Input: part model. Units: mm. Frame: model coordinates. A direction names the side the tool comes from. Give positions to 0.01 mm unless a question says otherwise; leave off trailing zeros. Order: outer loops, then holes, each group sorted by start corner. A loop starts at its lowest first (then second) coordinate and runs counter-clockwise, first axis right, second up. Notation, with made-up numbers: (87.5, 67.5) -> (135.5, 67.5) arc R8 cw to (135.5, 80.5) -> close; hole circle Ø11 at (72, 13). An arc over 180 degrees is marked (long way). Use a Markdown table: item, result. Add a question column.
from build123d import *

# Parameters (mm, degrees)
SKIZZE1_R                                            = 52.5
AUFSATZ_LINEAR_AUSTRAGEN1_DEPTH                      = 10
SKIZZE2_R                                            = 40
AUFSATZ_LINEAR_AUSTRAGEN3_DEPTH                      = 5
SKIZZE5_OUTSIDE_W                                    = 136.85
SKIZZE5_OUTSIDE_H                                    = 136.85
SKIZZE5_OUTSIDE_R                                    = 35
SCHNITT_LINEAR_AUSTRAGEN1_DEPTH                      = 5
SKIZZE6_R                                            = 38
AUFSATZ_LINEAR_AUSTRAGEN4_DEPTH                      = 5
SCHNITT_LINEAR_START                                 = -5
SKIZZE7_R                                            = 34.75
SCHNITT_LINEAR_AUSTRAGEN2_DEPTH                      = 10
SKIZZE10_R                                           = 25
SCHNITT_LINEAR_AUSTRAGEN4_DEPTH                      = 10
STIRNSENKUNG_F_R_M5_ZYLINDERSCHRAUBE_MIT_D           = 5.5
STIRNSENKUNG_F_R_M5_ZYLINDERSCHRAUBE_MIT_CBORE_D     = 10
STIRNSENKUNG_F_R_M5_ZYLINDERSCHRAUBE_MIT_CBORE_DEPTH = 5.4
KREISMUSTER4_COUNT                                   = 6
SKIZZE16_R                                           = 39
SKIZZE16_R_2                                         = 38
O_RING_NUT_DEPTH                                     = 1
SKIZZE17_R                                           = 40.85
SKIZZE17_R_2                                         = 38
SCHNITT_LINEAR_AUSTRAGEN5_DEPTH                      = 1.45
VERRUNDUNG1_R                                        = 0.3


with BuildPart() as part:
    # Skizze1 → Aufsatz-Linear austragen1 (new body)
    with BuildSketch(Plane.XY):
        Circle(SKIZZE1_R)
    extrude(amount=AUFSATZ_LINEAR_AUSTRAGEN1_DEPTH)

    # Skizze2 → Aufsatz-Linear austragen3 (add)
    with BuildSketch(Plane.XY):
        Circle(SKIZZE2_R)
    extrude(amount=-AUFSATZ_LINEAR_AUSTRAGEN3_DEPTH)

    # Skizze5 outside → Schnitt-Linear austragen1 (cut)
    with BuildSketch(Plane.XY):
        Rectangle(SKIZZE5_OUTSIDE_W, SKIZZE5_OUTSIDE_H)
        Circle(SKIZZE5_OUTSIDE_R, mode=Mode.SUBTRACT)
    extrude(amount=-SCHNITT_LINEAR_AUSTRAGEN1_DEPTH, mode=Mode.SUBTRACT)

    # Skizze6 → Aufsatz-Linear austragen4 (add)
    with BuildSketch(Plane.XY):
        Circle(SKIZZE6_R)
    extrude(amount=-AUFSATZ_LINEAR_AUSTRAGEN4_DEPTH)

    # Skizze7 → Schnitt-Linear austragen2 (cut)
    with BuildSketch(Plane.XY.offset(SCHNITT_LINEAR_START)):
        Circle(SKIZZE7_R)
    extrude(amount=SCHNITT_LINEAR_AUSTRAGEN2_DEPTH, mode=Mode.SUBTRACT)

    # Skizze10 → Schnitt-Linear austragen4 (cut)
    with BuildSketch(Plane.XY):
        Circle(SKIZZE10_R)
    extrude(amount=SCHNITT_LINEAR_AUSTRAGEN4_DEPTH, mode=Mode.SUBTRACT)

    # Stirnsenkung f_r M5 Zylinderschraube mit (through all)
    with Locations(Plane.XY.offset(10)):
        with Locations((0, -44)):
            stirnsenkung_f_r_m5_zylinderschraube_mit = CounterBoreHole(STIRNSENKUNG_F_R_M5_ZYLINDERSCHRAUBE_MIT_D / 2, STIRNSENKUNG_F_R_M5_ZYLINDERSCHRAUBE_MIT_CBORE_D / 2, STIRNSENKUNG_F_R_M5_ZYLINDERSCHRAUBE_MIT_CBORE_DEPTH)

    # Kreismuster4: Stirnsenkung f_r M5 Zylinderschraube mit ×6 about axis
    kreismuster4_axis = Axis((0, 0, 0), (0, 0, 1))
    for i in range(1, KREISMUSTER4_COUNT):
        add(stirnsenkung_f_r_m5_zylinderschraube_mit.rotate(kreismuster4_axis, i * 360 / KREISMUSTER4_COUNT), mode=Mode.SUBTRACT)

    # Skizze16 → o ring nut (cut)
    with BuildSketch(Plane(origin=(0, 0, 0), x_dir=(-1, 0, 0), z_dir=(0, 0, -1))):
        Circle(SKIZZE16_R)
        with Locations(Location((0, 0, 0), (0, 0, 180))):  # turned: the seam where the file's is
            Circle(SKIZZE16_R_2, mode=Mode.SUBTRACT)
    extrude(amount=-O_RING_NUT_DEPTH, mode=Mode.SUBTRACT)

    # Skizze17 → Schnitt-Linear austragen5 (cut)
    with BuildSketch(Plane(origin=(0, 0, 0), x_dir=(-1, 0, 0), z_dir=(0, 0, -1))):
        Circle(SKIZZE17_R)
        with Locations(Location((0, 0, 0), (0, 0, 180))):  # turned: the seam where the file's is
            Circle(SKIZZE17_R_2, mode=Mode.SUBTRACT)
    extrude(amount=-SCHNITT_LINEAR_AUSTRAGEN5_DEPTH, mode=Mode.SUBTRACT)

    # Verrundung1
    verrundung1_edges = [part.edges().sort_by_distance(p)[0] for p in [
        (40.85, 0, 1.45),
        (-38, 0, 1.45),
    ]]
    fillet(verrundung1_edges, radius=VERRUNDUNG1_R)


solid = part.part
Q1. Section query A-A (y = 0). Return loops of the section in (x, z), plus the area to 3 significant figures.
Q2. Access query for faces 5 (the cylindrical face through (17.535, -33.713, -1.882)), 6 (the cylindrical face through (-0.358, 41.273, 2.268)), 7 (the flat face through (41, -21, 4.6)). Directions: +Z, -Z, +X, -X, +Y, -Y. A direction counts if a zero-diameter tool reaches every point of the face in a straight line with its end or side. Return the directions, or none.
Q3. Ray query, line 1 (Y direction, x = 0, z = 7.7); line 2 (Y direction, x = -1, z = 4.5); line 3 (Z direction, x = -31, y = 1). Return the intervals inside material, ascending.
Q4. Section query B-B (y = 44). Return loops of the section in (x, z).
Q5. First-contact query: pin 1 (5 mm diameter, centred on y = -34.5, z = 1, fed in from -X); pin 2 (3.5 mm diameter, centred on x = -38.11, y = 22, fed in from -Z); pin 3 (5 mm diameter, centred on x = -37, y = 21.5, fed in from +Z); pin 4 (10 mm diameter, centred on x = 8.5, y = 20.5, fed in from -Z). Flat tips, straight axial feed; report the tip coordinate or a pass-through.
Q6. Draft query along Y for faces 1 (the cylindrical face through (50.076, 15.77, 4.93)), 2 (the cylindrical face through (-35.92, 20.33, 2.27)), 3 (the cylindrical face through (-38.756, 26.957, 7.338)), 4 (the flat face through (17, -31, -5)). Return one class per face: +Y half, -Y half, draft (parallel to the pull), parting line (faces both ways), or undercut.
Q7. Section query C-C (x = 0). Give the number of separate pieces and of enclosed holes in the cut face, plus the area to 3 significant figures.
Solution:
| question | item | result |
|---|---|---|
| 1 | outline | (-52.5, 0) -> (-40.85, 0) -> (-40.85, 1.15) arc R0.3 cw to (-40.55, 1.45) -> (-38.3, 1.45) arc R0.3 cw to (-38, 1.15) -> (-38, -5) -> (-34.75, -5) -> (-34.75, 5) -> (-25, 5) -> (-25, 10) -> (-52.5, 10) -> close; (25, 5) -> (34.75, 5) -> (34.75, -5) -> (38, -5) -> (38, 1.15) arc R0.3 cw to (38.3, 1.45) -> (40.55, 1.45) arc R0.3 cw to (40.85, 1.15) -> (40.85, 0) -> (52.5, 0) -> (52.5, 10) -> (25, 10) -> close |
| 1 | area | 477 mm² |
| 2 | face 5 | -Z |
| 2 | face 6 | +Z, -Z |
| 2 | face 7 | +Z |
| 3 | line 1 | y = -52.5 to -49, -39 to -25, 25 to 39, 49 to 52.5 |
| 3 | line 2 | y = -52.49 to -46.56, -41.44 to -34.74, 34.74 to 41.44, 46.56 to 52.49 |
| 3 | line 3 | z = 5 to 10 |
| 4 | outline | (-28.64, 0) -> (-2.75, 0) -> (-2.75, 4.6) -> (-5, 4.6) -> (-5, 10) -> (-28.64, 10) -> close; (2.75, 0) -> (28.64, 0) -> (28.64, 10) -> (5, 10) -> (5, 4.6) -> (2.75, 4.6) -> close |
| 5 | pin 1 | stops at x = -41.62 |
| 5 | pin 2 | passes through |
| 5 | pin 3 | stops at z = 4.6 |
| 5 | pin 4 | stops at z = 5 |
| 6 | face 1 | parting line |
| 6 | face 2 | undercut |
| 6 | face 3 | undercut |
| 6 | face 4 | draft |
| 7 | separate pieces | 4 |
| 7 | enclosed holes | 0 |
| 7 | area | 318 mm² |
